from build123d import *

# Parameters (mm, degrees)
F0_W     = 1219.2
F0_H     = 914.4
F1_DEPTH = 457.2
F2_W     = 1078.8844227791
F2_H     = 796.030819416
F3_DEPTH = 381
F4_R     = 73.4303316823
F5_DEPTH = 127
F6_W     = 38.5419428349
F6_H     = 398.015409708
F6_W_2   = 34.6445441246
F6_H_2   = 404.1308164597
F6_W_3   = 42.8168773651
F6_H_3   = 796.030819416
F6_W_4   = 35.4440659285
F7_DEPTH = 50


with BuildPart() as f1:
    # F0 (on Top) → F1 (new body)
    with BuildSketch(Plane.XY):
        with Locations((609.6, -457.2)):
            Rectangle(F0_W, F0_H)
    extrude(amount=F1_DEPTH)

    # F2 (on face) → F3 (cut)
    with BuildSketch(Plane.XY.offset(457.2)):
        with Locations((606.4463555813, -458.0872356892)):
            Rectangle(F2_W, F2_H)
    extrude(amount=-F3_DEPTH, mode=Mode.SUBTRACT)

    # F4 (on face) → F5 (cut)
    with BuildSketch(Plane(origin=(0, 0, 0), x_dir=(0, -1, 0), z_dir=(-1, 0, 0))):
        with Locations((457.2, 233.6474359035)):
            Circle(F4_R)
    extrude(amount=-F5_DEPTH, mode=Mode.SUBTRACT)

    # F6 (on face) → F7 (join)
    with BuildSketch(Plane.XY.offset(76.2)):
        with Locations((466.0627692938, -259.0795308352)):
            Rectangle(F6_W, F6_H)
        with Locations((708.6218893528, -654.0372371674)):
            Rectangle(F6_W_2, F6_H_2)
        with Locations((918.1770086288, -458.0872356892)):
            Rectangle(F6_W_3, F6_H_3)
        with Locations((252.6499405503, -458.0872356892)):
            Rectangle(F6_W_4, F6_H_3)
    extrude(amount=F7_DEPTH)


solid = f1.part
Geometry check sheet. Reference: the model listing, model coordinates, mm. A direction names the side the tool comes from. Round coordinates to 2 decimals unless told otherwise and drop trailing zeros. Order: outer loops, then holes, each group sorted by start corner. A loop starts at its lowest first (then second) coordinate and runs counter-clockwise, first axis right, second up. Notation, with made-up numbers: M 15.25,54 L 47.25,54 A30 cw 47.25,86 Z; hole C -3.75,23 d6. An arc over 180 degrees is marked long. Answer in a Markdown table with one row per item.
(1) Scan lines: probe 1 along X at (y, z) = (-74.5, 427); probe 2 along Y at (x, z) = (181, 407.5); probe 3 along Z at (x, y) = (31, -457). Record each from-to range of solid material in increasing order. Write a range as from..to.
Responses:
| item | result |
|---|---|
| probe 1 | x = 0..67, 1145.89..1219.2 |
| probe 2 | y = -914.4..-856.1, -60.07..0 |
| probe 3 | z = 0..160.22, 307.08..457.2 |
(2) Go/stop test with flat-tipped pins: P1, Ø12, axis at x = 682, y = -558, coming from the +Z side; P2, Ø10, axis at x = 708, y = -574.5, coming from the +Z side. Record where each tip stops, or that it passes through.
Responses:
| item | result |
|---|---|
| P1 | stops at z = 76.2 |
| P2 | stops at z = 126.2 |
(3) Sectioned sample at A-A, the plane y = -514.5. Record the cut outline in (x, z), and give its area (3 significant figures).
Responses:
| item | result |
|---|---|
| outline | M 0,0 L 1219.2,0 L 1219.2,457.2 L 1145.89,457.2 L 1145.89,76.2 L 939.59,76.2 L 939.59,126.2 L 896.77,126.2 L 896.77,76.2 L 725.94,76.2 L 725.94,126.2 L 691.3,126.2 L 691.3,76.2 L 270.37,76.2 L 270.37,126.2 L 234.93,126.2 L 234.93,76.2 L 67,76.2 L 67,187.73 L 0,187.73 Z; M 0,279.57 L 67,279.57 L 67,457.2 L 0,457.2 Z |
| area | 146,000 mm² |
(4) Sectioned sample at B-B, the plane x = 1030.5. Record the cut outline in (y, z), and give its area (3 significant figures).
Responses:
| item | result |
|---|---|
| outline | M -914.4,0 L 0,0 L 0,457.2 L -60.07,457.2 L -60.07,76.2 L -856.1,76.2 L -856.1,457.2 L -914.4,457.2 Z |
| area | 115,000 mm² |
(5) Sectioned sample at D-D, the plane y = -704. Record the cut outline in (x, z), and give its area (3 significant figures).
Responses:
| item | result |
|---|---|
| outline | M 0,0 L 1219.2,0 L 1219.2,457.2 L 1145.89,457.2 L 1145.89,76.2 L 939.59,76.2 L 939.59,126.2 L 896.77,126.2 L 896.77,76.2 L 725.94,76.2 L 725.94,126.2 L 691.3,126.2 L 691.3,76.2 L 270.37,76.2 L 270.37,126.2 L 234.93,126.2 L 234.93,76.2 L 67,76.2 L 67,457.2 L 0,457.2 Z |
| area | 152,000 mm² |
(6) Draft check along X on faces 4 (the face through (1219.2, -464, 225)), 5 (the face through (939.585, -464, 101)), 6 (the face through (601, -451, 0)). Enter one of: released by +X, released by -X, zero draft, split by the parting line, or undercut.
Responses:
| item | result |
|---|---|
| face 4 | released by +X |
| face 5 | undercut |
| face 6 | zero draft |
(7) Tool access check on faces 1 (the face through (67.004, -464, 312)), 2 (the face through (33.03, -525.03, 205.52)), 3 (the face through (607, -49, 457.2)). Record the directions out of +Z, -Z, +X, -X, +Y, -Y that give a thin tool (end or side, any length) a straight path to the whole face; none if there is none.
Responses:
| item | result |
|---|---|
| face 1 | +Z |
| face 2 | -X |
| face 3 | +Z, +X, -X, +Y, -Y |
(8) Sectioned sample at C-C, the plane y = -310.5. Record the cut outline in (x, z).
Responses:
| item | result |
|---|---|
| outline | M 0,0 L 1219.2,0 L 1219.2,457.2 L 1145.89,457.2 L 1145.89,76.2 L 939.59,76.2 L 939.59,126.2 L 896.77,126.2 L 896.77,76.2 L 485.33,76.2 L 485.33,126.2 L 446.79,126.2 L 446.79,76.2 L 270.37,76.2 L 270.37,126.2 L 234.93,126.2 L 234.93,76.2 L 67,76.2 L 67,457.2 L 0,457.2 Z |
